The figure shows three views and two pictorial views of one solid part (mm, origin at its lowest corner). Answer the questions. A direction names the side the tool comes from. Coordinates: 2 decimals unless noted, no trailing zeros. Loops run counter-clockwise (first coordinate to the right, second up) from the corner with the lowest first, then second, coordinate; pieces in that order, holes last. Notation, with made-up numbers: M -2.75,76.25 L 41.25,76.25 A25 cw 41.25,111.25 Z; hole C -4.5,-14.75 d11. An arc over 180 degrees is marked long. Answer as a JSON object with one key per item and string values. Group by question number.
1. Determine the mould class of the marked faces 1, 2 and 3 for opening direction Z: released by +Z, released by -Z, zero draft, split by the parting line, or undercut.
2. A cutting plane is placed at D-D on x = 4. Give the vertices of the cut face in (y, z).
3. A cutting plane is placed at A-A on x = 11.5. Give the vertices of the cut face in (y, z), and give its area (3 significant figures).
4. Straight lines are drawn through the part: L1, parallel to X at y = 2.35, z = 4; L2, parallel to Z at x = 46, y = 3.25; L3, parallel to X at y = 0.3, z = 13. For each, find the intervals that lie inside material, in ascending order.
5. A cutting plane is placed at B-B on y = 2.95. Give the vertices of the cut face in (x, z).
6. A cutting plane is placed at C-C on z = 4. Give the vertices of the cut face in (x, y).
7. For the marked faces 4 and 5, determine the directions among +Z, -Z, +X, -X, +Y, -Y from which every point of the face is accessible in a straight line to the end or side of a thin tool.
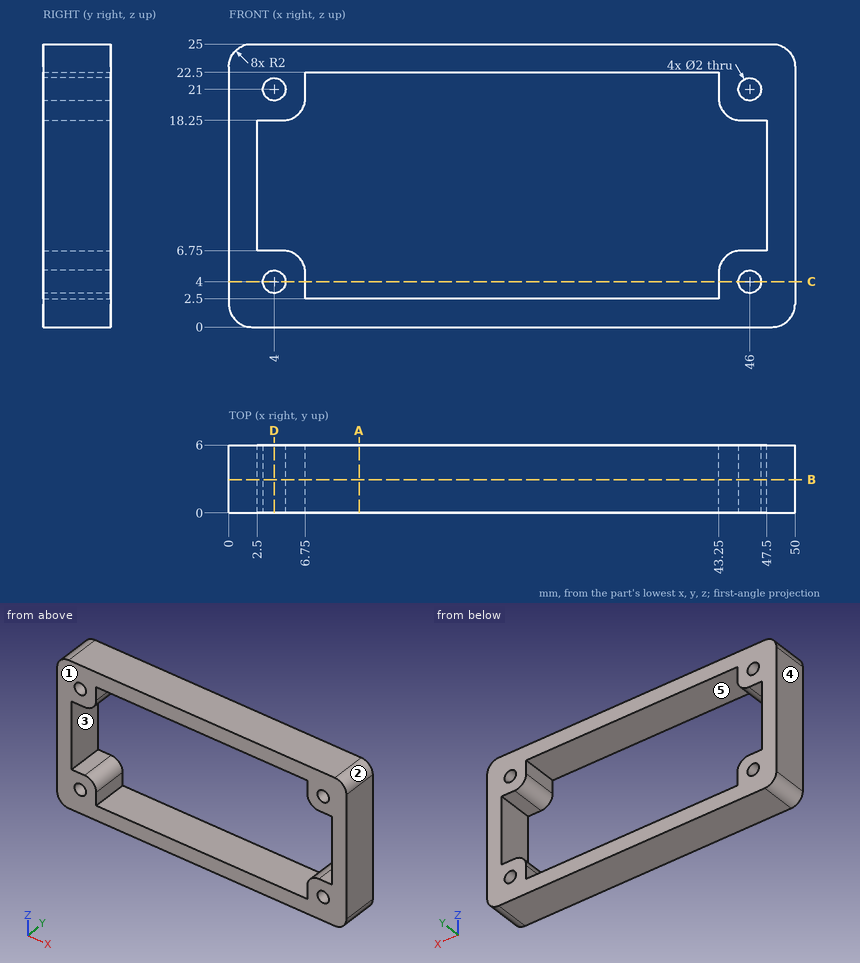
From the geometry:
{
 "1": {"face 1": "zero draft", "face 2": "released by +Z", "face 3": "undercut"},
 "2": {"outline": "M 0,0 L 6,0 L 6,3 L 0,3 Z; M 0,5 L 6,5 L 6,6.75 L 0,6.75 Z; M 0,18.25 L 6,18.25 L 6,20 L 0,20 Z; M 0,22 L 6,22 L 6,25 L 0,25 Z"},
 "3": {"outline": "M 0,0 L 6,0 L 6,2.5 L 0,2.5 Z; M 0,22.5 L 6,22.5 L 6,25 L 0,25 Z", "area": "30.0 mm²"},
 "4": {"L1": "x = 0 to 3, 5 to 6.75, 43.25 to 45, 47 to 50", "L2": "z = 0 to 3, 5 to 6.75, 18.25 to 20, 22 to 25", "L3": "x = 0 to 2.5, 47.5 to 50"},
 "5": {"outline": "M 0,2 A2 ccw 2,0 L 48,0 A2 ccw 50,2 L 50,23 A2 ccw 48,25 L 2,25 A2 ccw 0,23 Z; hole M 2.5,6.75 L 4.75,6.75 A2 cw 6.75,4.75 L 6.75,2.5 L 43.25,2.5 L 43.25,4.75 A2 cw 45.25,6.75 L 47.5,6.75 L 47.5,18.25 L 45.25,18.25 A2 cw 43.25,20.25 L 43.25,22.5 L 6.75,22.5 L 6.75,20.25 A2 cw 4.75,18.25 L 2.5,18.25 Z; hole C 4,4 d2; hole C 4,21 d2; hole C 46,4 d2; hole C 46,21 d2"},
 "6": {"outline": "M 0,0 L 3,0 L 3,6 L 0,6 Z; M 5,0 L 6.75,0 L 6.75,6 L 5,6 Z; M 43.25,0 L 45,0 L 45,6 L 43.25,6 Z; M 47,0 L 50,0 L 50,6 L 47,6 Z"},
 "7": {"face 4": "+Z, -Z, -X, +Y, -Y", "face 5": "+Y, -Y"}
}
